Part model, mm, in its own coordinate system. Round coordinates to 2 decimals unless told otherwise and drop trailing zeros. Loops run counter-clockwise (first coordinate to the right, second up) from the corner with the lowest first, then second, coordinate; pieces in that order, holes last. Notation, with made-up numbers: M 40,-27.75 L 86,-27.75 A29 cw 86,-4.75 Z; hole C 47,46.25 d11. An arc over 180 degrees is marked long. Put each result on its own line as item: value. Start each with the question number.
1) Slice it at B-B on z = 15. Give the cut face in (x, y), then the cut area to 3 significant figures.
2) Drop flat-ended pins along their axis: pin 1 Ø7 at (x, z) = (5.5, -15) entering from +Y; pin 2 Ø8.5 at (x, z) = (5.5, 15) entering from +Y; pin 3 Ø8 at (x, z) = (5.5, 14.5) entering from +Y; pin 4 Ø3 at (x, z) = (5.5, 15) entering from -Y. Give the stop position or say it passes through.
3) Probe line 1 along X through (y, z) = (4.3, -15); line 2 along Z through (x, y) = (-5.5, 1.45); line 3 along Z through (x, y) = (5.5, 4.9). List the from-to ranges inside material, lowest first.
4) Slice it at A-A on x = -5.5. Give the cut face in (y, z), then the cut area to 3 significant figures.
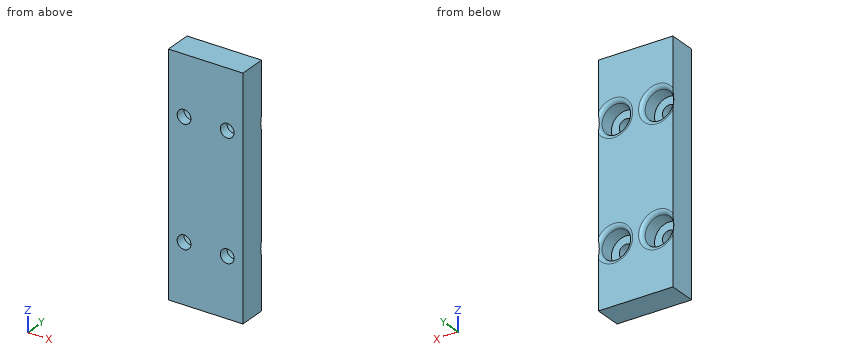
Autodesk Inventor part; units mm, degrees
ref_plane "YZ Plane" through (0, 0, 0) normal (1, 0, 0) x (0, 1, 0)
ref_plane "XZ Plane" through (0, 0, 0) normal (0, 1, 0) x (-1, 0, 0)
ref_plane "XY Plane" through (0, 0, 0) normal (0, 0, 1) x (1, 0, 0)
sketch "Esquisse1" plane through (0, 0, 0) normal (0, 1, 0) x (-1, 0, 0)
  line L0 (-9.5, 30) -> (9.5, 30)
  line L1 (9.5, 30) -> (9.5, -30)
  line L2 (9.5, -30) -> (-9.5, -30)
  line L3 (-9.5, -30) -> (-9.5, 30)
  line L4 (-9.5, 30) -> (9.5, -30) construction
  line L5 (9.5, 30) -> (-9.5, -30) construction
  circle A0 centre (5.5, 15) radius 1.75
  circle A1 centre (5.5, -15) radius 1.75
  line L6 (0, 32.5338) -> (0, -37.7206)
  circle A2 centre (-5.5, 15) radius 1.75
  circle A3 centre (-5.5, -15) radius 1.75
  point P0 (0, 0)
  dimension "d0" = 19
  dimension "d1" = 60
  dimension "d2" = 15
  dimension "d3" = 15
  dimension "d4" = 3.5
  dimension "d11" = 4
  dimension "d12" = 4
extrude "Extrusion1" add sketch "Esquisse1" along normal blind 7
sketch "Esquisse2" plane through (0, 7, 0) normal (0, 1, 0) x (1, 0, 0)
  circle A0 centre (-5.5, -15) radius 1.75
  circle A1 centre (-5.5, -15) radius 3.75
  circle A2 centre (-5.5, 15) radius 1.75
  circle A3 centre (-5.5, 15) radius 3.75
  line L0 (0, -33.1726) -> (0, 42.5186)
  circle A4 centre (5.5, -15) radius 1.75
  circle A5 centre (5.5, -15) radius 3.75
  circle A6 centre (5.5, 15) radius 1.75
  circle A7 centre (5.5, 15) radius 3.75
  point P0 (0, 0)
  dimension "d7" = 7.5
extrude "Extrusion2" cut sketch "Esquisse2" against normal blind 4.5 contours A1 | A3 | A5 | A6 | A7
fillet "Congé2" radius 1 4 edges at (-9.25, 7, -15) (1.75, 7, -15) (-9.25, 7, 15) (1.75, 7, 15)
properties part number "attache_cadre"
Recorded:
1. outline: M -9.5,0 L -7.25,0 L -7.25,2.5 L -9.25,2.5 L -9.25,6 A1 ccw -9.5,6.66 Z; M -3.75,0 L 3.75,0 L 3.75,2.5 L 1.75,2.5 L 1.75,6 A1 ccw 0.75,7 L -0.75,7 A1 ccw -1.75,6 L -1.75,2.5 L -3.75,2.5 Z; M 7.25,0 L 9.5,0 L 9.5,6.66 A1 ccw 9.25,6 L 9.25,2.5 L 7.25,2.5 Z
1. area: 47.3 mm2
2. pin 1: stops at y = 2.5
2. pin 2: stops at y = 6.87
2. pin 3: stops at y = 6.97
2. pin 4: passes through
3. line 1: x = -9.5 to -9.25, -1.75 to 1.75, 9.25 to 9.5
3. line 2: z = -30 to -16.75, -13.25 to 13.25, 16.75 to 30
3. line 3: z = -30 to -18.75, -11.25 to 11.25, 18.75 to 30
4. outline: M 0,-30 L 7,-30 L 7,-19.75 A1 ccw 6,-18.75 L 2.5,-18.75 L 2.5,-16.75 L 0,-16.75 Z; M 0,-13.25 L 2.5,-13.25 L 2.5,-11.25 L 6,-11.25 A1 ccw 7,-10.25 L 7,10.25 A1 ccw 6,11.25 L 2.5,11.25 L 2.5,13.25 L 0,13.25 Z; M 0,16.75 L 2.5,16.75 L 2.5,18.75 L 6,18.75 A1 ccw 7,19.75 L 7,30 L 0,30 Z
4. area: 334 mm2
